Part print with two shaded views. Sizes in mm from the minimum x, y, z corner. A direction names the side the tool comes from. Give positions to 0.01 mm unless a question says otherwise; leave off trailing zeros. Write each loop counter-clockwise with the first axis right and the second up, starting at its lowest first coordinate (ties: lowest second). Pieces come first, ordered by that corner, then holes.
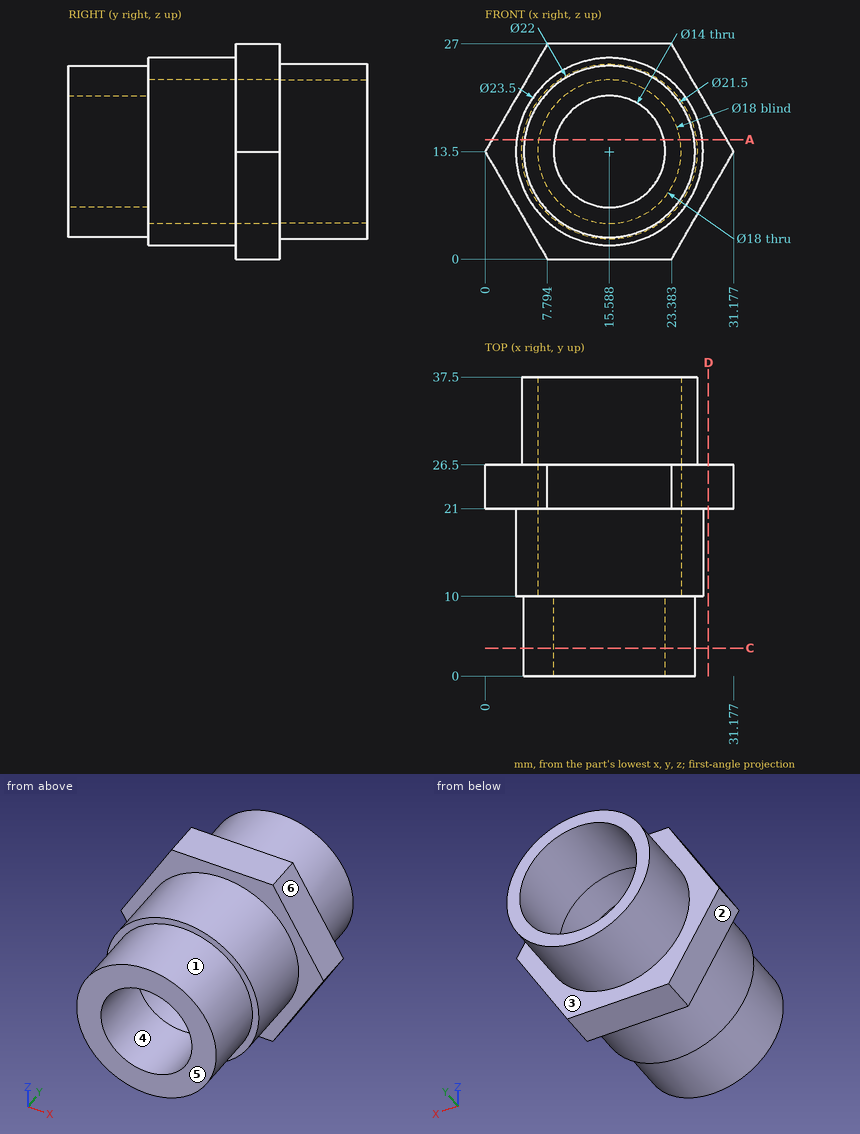
(1) Saw through at A-A, the plane z = 15. List the corners of the cut face in (x, y) (1 decimal).
(2) Mould opens along X. For the marked faces 4, 5 and 6 say: +X half, -X half, draft (parallel to the pull), parting line (faces both ways), or undercut.
(3) Saw through at C-C, the plane y = 3.5. List the corners of the cut face in (x, z), plus the area to 3 significant figures.
(4) Probe line 1 (X direction, y = 2.25, z = 13.5); line 2 (X direction, y = 14.75, z = 13.5); line 3 (Y direction, x = 10, z = 23.5). List the from-to ranges inside material, lowest first.
(5) Drop flat-ended pins along their axis: pin 1 (5 mm diameter, centred on x = 19.5, y = 16.5, fed in from -Z) (1 decimal); pin 2 (12 mm diameter, centred on y = 8.5, z = 22.5, fed in from -X); pin 3 (1 mm diameter, centred on y = 23, z = 4.5, fed in from +X); pin 4 (1.5 mm diameter, centred on x = 26, z = 14.5, fed in from -Y). Give the stop position or say it passes through.
(6) 3-axis set-ups, long thin cutter, end or side, ignore diameter. For the marked faces 1, 2 and 3: which of +Z, -Z, +X, -X, +Y, -Y reach the whole face in a straight line?
(7) Saw through at D-D, the plane x = 28. List the corners of the cut face in (y, z).
Computed values:
1. outline: (0.9, 21) - (3.9, 21) - (3.9, 10) - (4.9, 10) - (4.9, 0) - (8.8, 0) - (8.8, 10) - (6.7, 10) - (6.7, 37.5) - (4.7, 37.5) - (4.7, 26.5) - (0.9, 26.5) - close; (22.4, 0) - (26.2, 0) - (26.2, 10) - (27.2, 10) - (27.2, 21) - (30.3, 21) - (30.3, 26.5) - (26.5, 26.5) - (26.5, 37.5) - (24.5, 37.5) - (24.5, 10) - (22.4, 10) - close
2. face 4: undercut
2. face 5: draft
2. face 6: +X half
3. outline: circle Ø21.5 at (15.59, 13.5); hole circle Ø14 at (15.59, 13.5)
3. area: 209 mm2
4. line 1: x = 4.84 to 8.59, 22.59 to 26.34
4. line 2: x = 3.84 to 6.59, 24.59 to 27.34
4. line 3: y = 10 to 26.5
5. pin 1: stops at z = 1.8
5. pin 2: stops at x = 4.28
5. pin 3: stops at x = 26.27
5. pin 4: stops at y = 0
6. face 1: -Y
6. face 2: -Z, -X, +Y, -Y
6. face 3: +Y
7. outline: (21, 8) - (26.5, 8) - (26.5, 19) - (21, 19) - close
